from build123d import *

# Parameters (mm, degrees)
PAD001_DEPTH      = 15
PAD001_DEPTH_BACK = 15
SKETCH014_W       = 8
SKETCH014_H       = 6
POCKET_DEPTH      = 11
SKETCH013_R       = 1.4
SKETCH013_R_2     = 1.75
POCKET001_DEPTH   = 17
SKETCH012_R       = 5.15
POCKET002_DEPTH   = 43.001
SKETCH007_R       = 1.75
POCKET003_DEPTH   = 17.001
SKETCH008_W       = 8.907674
SKETCH008_H       = 16
SKETCH008_W_2     = 9.43002
SKETCH008_H_2     = 13.41794
POCKET004_DEPTH   = 31
SKETCH018_R       = 3
POCKET005_DEPTH   = 55.001
SKETCH021_W       = 22.157055
SKETCH021_H       = 18.106247
POCKET006_DEPTH   = 44
SKETCH015_W       = 50.47
SKETCH015_H       = 40
POCKET007_DEPTH   = 3
FILLET_R          = 3
FILLET001_R       = 1
FILLET002_R       = 2
FILLET003_R       = 1
FILLET004_R       = 1
FILLET005_R       = 1
FILLET006_R       = 1
FILLET007_R       = 5
FILLET008_R       = 1
FILLET009_R       = 0.8
FILLET010_R       = 0.5
FILLET011_R       = 0.5
FILLET012_R       = 0.5
FILLET013_R       = 1


with BuildPart() as part:
    # Sketch005 → Pad001 (new body, two sides)
    with BuildSketch(Plane.YZ) as pad001_sk:
        Polygon((0, -20), (0, 17), (3, 17), (3, 23), (-25, 23), (-25, 13), (-14, 13), (-14, -20), align=None)
    extrude(amount=PAD001_DEPTH)
    extrude(pad001_sk.sketch, amount=-PAD001_DEPTH_BACK)

    # Sketch014 (on Face5 of Pad001) → Pocket (cut)
    with BuildSketch(Plane(origin=(0, -25, 0), x_dir=(0, 0, -1), z_dir=(0, -1, 0))):
        with Locations((-15, -8)):
            Rectangle(SKETCH014_W, SKETCH014_H)
    extrude(amount=-POCKET_DEPTH, mode=Mode.SUBTRACT)

    # Sketch013 → Pocket001 (cut)
    with BuildSketch(Plane(origin=(0, 0, 35), x_dir=(0, -1, 0), z_dir=(0, 0, 1))):
        with Locations((4, -8)):
            Circle(SKETCH013_R)
        with Locations((22, -8)):
            Circle(SKETCH013_R_2)
    extrude(amount=-POCKET001_DEPTH, mode=Mode.SUBTRACT)

    # Sketch012 (on Face4 of Pad001) → Pocket002 (cut, through all)
    with BuildSketch(Plane(origin=(0, 0, 23), x_dir=(0, -1, 0), z_dir=(0, 0, 1))):
        with Locations((13, -8)):
            Circle(SKETCH012_R)
    extrude(amount=-POCKET002_DEPTH, mode=Mode.SUBTRACT)

    # Sketch007 → Pocket003 (cut, through all)
    with BuildSketch(Plane(origin=(0, -14, 0), x_dir=(0, 0, -1), z_dir=(0, -1, 0))):
        with Locations((-6, 10)):
            Circle(SKETCH007_R)
        with Locations((14, 10)):
            Circle(SKETCH007_R)
        with Locations((-6, -10)):
            Circle(SKETCH007_R)
        with Locations((14, -10)):
            Circle(SKETCH007_R)
    extrude(amount=-POCKET003_DEPTH, mode=Mode.SUBTRACT)

    # Sketch008 → Pocket004 (cut)
    with BuildSketch(Plane.YX.offset(20)):
        with Locations((-10.453837, -8)):
            Rectangle(SKETCH008_W, SKETCH008_H)
        with Locations((-10.71501, 10.872729)):
            Rectangle(SKETCH008_W_2, SKETCH008_H_2)
    extrude(amount=-POCKET004_DEPTH, mode=Mode.SUBTRACT)

    # Sketch018 → Pocket005 (cut, through all)
    with BuildSketch(Plane(origin=(0, 0, 35), x_dir=(0, -1, 0), z_dir=(0, 0, 1))):
        with Locations((25.735598, 1.909207)):
            Circle(SKETCH018_R)
    extrude(amount=-POCKET005_DEPTH, mode=Mode.SUBTRACT)

    # Sketch021 → Pocket006 (cut)
    with BuildSketch(Plane(origin=(0, 0, 23), x_dir=(0, -1, 0), z_dir=(0, 0, 1))):
        with Locations((17.078527, 11.053123)):
            Rectangle(SKETCH021_W, SKETCH021_H)
    extrude(amount=-POCKET006_DEPTH, mode=Mode.SUBTRACT)

    # Sketch015 → Pocket007 (cut)
    with BuildSketch(Plane.ZX):
        with Locations((-9.235, 0)):
            Rectangle(SKETCH015_W, SKETCH015_H)
    extrude(amount=-POCKET007_DEPTH, mode=Mode.SUBTRACT)

    # Fillet
    fillet_edges = [part.edges().sort_by_distance(p)[0] for p in [
        (-15, 3, 20),
        (-15, -25, 18),
        (15, 3, 20),
    ]]
    fillet(fillet_edges, radius=FILLET_R)

    # Fillet001
    fillet001_edges = [part.edges().sort_by_distance(p)[0] for p in [
        (15, -6, 17),
    ]]
    fillet(fillet001_edges, radius=FILLET001_R)

    # Fillet002
    fillet002_edges = [part.edges().sort_by_distance(p)[0] for p in [
        (2, -6, 1.5),
    ]]
    fillet(fillet002_edges, radius=FILLET002_R)

    # Fillet003
    fillet003_edges = [part.edges().sort_by_distance(p)[0] for p in [
        (2, -22.736972, 18),
        (-0.999211, -25, 18),
    ]]
    fillet(fillet003_edges, radius=FILLET003_R)

    # Fillet004
    fillet004_edges = [part.edges().sort_by_distance(p)[0] for p in [
        (-15, -6, -4.5),
    ]]
    fillet(fillet004_edges, radius=FILLET004_R)

    # Fillet005
    fillet005_edges = [part.edges().sort_by_distance(p)[0] for p in [
        (-15, -3, -2),
    ]]
    fillet(fillet005_edges, radius=FILLET005_R)

    # Fillet006
    fillet006_edges = [part.edges().sort_by_distance(p)[0] for p in [
        (15, -3, -2),
    ]]
    fillet(fillet006_edges, radius=FILLET006_R)

    # Fillet007
    fillet007_edges = [part.edges().sort_by_distance(p)[0] for p in [
        (0, -6, -4.5),
    ]]
    fillet(fillet007_edges, radius=FILLET007_R)

    # Fillet008
    fillet008_edges = [part.edges().sort_by_distance(p)[0] for p in [
        (-5, -25, 16),
    ]]
    fillet(fillet008_edges, radius=FILLET008_R)

    # Fillet009
    fillet009_edges = [part.edges().sort_by_distance(p)[0] for p in [
        (-11, -25, 16),
    ]]
    fillet(fillet009_edges, radius=FILLET009_R)

    # Fillet010
    fillet010_edges = [part.edges().sort_by_distance(p)[0] for p in [
        (0, -14, -4.5),
    ]]
    fillet(fillet010_edges, radius=FILLET010_R)

    # Fillet011
    fillet011_edges = [part.edges().sort_by_distance(p)[0] for p in [
        (2, -14, -3.5),
    ]]
    fillet(fillet011_edges, radius=FILLET011_R)

    # Fillet012
    fillet012_edges = [part.edges().sort_by_distance(p)[0] for p in [
        (-15, -14, 12),
    ]]
    fillet(fillet012_edges, radius=FILLET012_R)

    # Fillet013
    fillet013_edges = [part.edges().sort_by_distance(p)[0] for p in [
        (-13.05198, -14, 12),
        (-2.94802, -14, 12),
    ]]
    fillet(fillet013_edges, radius=FILLET013_R)


solid = part.part
Geometry check sheet. Reference: the model listing, model coordinates, mm. A direction names the side the tool comes from. Round coordinates to 2 decimals unless told otherwise and drop trailing zeros. Loops run counter-clockwise (first coordinate to the right, second up) from the corner with the lowest first, then second, coordinate; pieces in that order, holes last. Notation, with made-up numbers: (75, 13.5) -> (109, 13.5) arc R23 ccw to (109, 43.5) -> close; hole circle Ø7 at (-39, 5.5). An arc over 180 degrees is marked (long way). Answer as a JSON object with one key per item and string values. Group by question number.
Item 1: Cross-section at B-B, the plane x = 10. Record the cut outline in (y, z), plus the area to 3 significant figures.
Item 2: Release check for a two-part mould opening along X. For faces 1 (the face through (-15, -11, 16)), 2 (the face through (-2.549, -13.715, 12.014)), 3 (the face through (14.699, -3.285, -1.748)) record: pulls with the +X half, pulls with the -X half, needs draft (parallel to the pull), parting line crosses it, or undercut.
Item 3: Cross-section at A-A, the plane z = 6. Record the cut outline in (x, y).
Item 4: Depth check by flat-ended pin: pin 1 Ø3.5 at (x, z) = (0.5, -7) entering from -Y; pin 2 Ø3 at (x, z) = (-2, -13) entering from +Y; pin 3 Ø4 at (x, z) = (10, -14) entering from -Y; pin 4 Ø6 at (x, y) = (-8, -13) entering from -Z. Enter the tip coordinate at first touch or a pass-through.
Item 5: Cross-section at D-D, the plane z = -8. Record the cut outline in (x, y), plus the area to 3 significant figures.
Item 6: Set-up check for faces 4 (the face through (0, -12, -5)), 5 (the face through (-14.715, -3.301, -1.748)), 6 (the face through (-7, -20, 19)), 7 (the face through (-8.265, -4.521, 6.228)), 8 (the face through (0, -3, -2)): record each of +Z, -Z, +X, -X, +Y, -Y from which the full face is reachable in a straight line by a thin tool's end or side.
Item 7: Thickness scan on line 1 along X through (y, z) = (-4.55, 6); line 2 along X through (y, z) = (-4, 19.25); line 3 along Y through (x, z) = (4.75, -2.5). Record the ranges inside material, lowest first.
Item 8: Cross-section at C-C, the plane y = -9.75. Record the cut outline in (x, z) (3 decimals), plus the area to 3 significant figures.
Determined:
{
 "1": {"outline": "(-6, -20) -> (-3, -20) -> (-3, -15.75) -> (-6, -15.75) -> close; (-6, -12.25) -> (-3, -12.25) -> (-3, 4.25) -> (-6, 4.25) -> close; (-6, 7.75) -> (-3, 7.75) -> (-3, 16) -> (0, 16) -> (0, 17) -> (3, 17) -> (3, 23) -> (-6, 23) -> close", "area": "147 mm²"},
 "2": {"face 1": "pulls with the -X half", "face 2": "undercut", "face 3": "pulls with the +X half"},
 "3": {"outline": "(-15, -5) arc R1 ccw to (-14, -6) -> (-11.75, -6) -> (-11.75, -3) -> (-14, -3) arc R1 ccw to (-15, -4) -> close; (-8.25, -6) -> (-5, -6) arc R5 cw to (0, -11) -> (0, -13.5) arc R0.5 ccw to (0.5, -14) -> (1.5, -14) arc R0.5 ccw to (2, -13.5) -> (2, -8) arc R2 cw to (4, -6) -> (8.25, -6) -> (8.25, -3) -> (-8.25, -3) -> close; (11.75, -6) -> (14, -6) arc R1 ccw to (15, -5) -> (15, -4) arc R1 ccw to (14, -3) -> (11.75, -3) -> close"},
 "4": {"pin 1": "stops at y = -14", "pin 2": "stops at y = -3", "pin 3": "stops at y = -6", "pin 4": "passes through"},
 "5": {"outline": "(-15, -5) arc R1 ccw to (-14, -6) -> (-5, -6) arc R5 cw to (0, -11) -> (0, -13.5) arc R0.5 ccw to (0.5, -14) -> (1.5, -14) arc R0.5 ccw to (2, -13.5) -> (2, -8) arc R2 cw to (4, -6) -> (14, -6) arc R1 ccw to (15, -5) -> (15, -4) arc R1 ccw to (14, -3) -> (-14, -3) arc R1 ccw to (-15, -4) -> close", "area": "111 mm²"},
 "6": {"face 4": "-Z, -X, -Y", "face 5": "-Z, -X, +Y", "face 6": "-Z, -Y", "face 7": "+Y, -Y", "face 8": "-Z, +X, -X, +Y"},
 "7": {"line 1": "x = -15 to -11.75, -8.25 to 8.25, 11.75 to 15", "line 2": "x = -15 to -9.4, -6.6 to 15", "line 3": "y = -6 to -3"},
 "8": {"outline": "(-15, 11) -> (-11.995, 11) -> (-11.995, 23) -> (-15, 23) -> close; (-4.005, 11) -> (-0.159, 11) -> (-0.159, -20) -> (2, -20) -> (2, 23) -> (-4.005, 23) -> close", "area": "175 mm²"}
}
